Build history of the part. All positions in model axes, mm. A direction names the side the tool comes from. Round coordinates to 2 decimals unless told otherwise and drop trailing zeros. Loops run counter-clockwise (first coordinate to the right, second up) from the corner with the lowest first, then second, coordinate; pieces in that order, holes last.
Autodesk Inventor part; units mm, degrees
ref_plane "Work Plane2" through (0, 0, 11.8) normal (0, 0, 1) x (1, 0, 0)
ref_plane "Work Plane1" through (0, 0, 21.8) normal (0, 1, 0) x (0, 0, 1)
ref_plane "YZ Plane" through (0, 0, 0) normal (1, 0, 0) x (0, 1, 0)
sketch "Sketch1" plane through (0, 0, 0) normal (0, 0, 1) x (1, 0, 0)
  arc A0 (4.825, 0) -> (-4.825, 0) centre (0, 0) ccw
  line L0 (4.825, 0) -> (4.825, -3.775)
  line L1 (4.825, -3.775) -> (-4.825, -3.775)
  line L2 (-4.825, -3.775) -> (-4.825, 0)
  dimension "d0" = 9.65
  dimension "d2" = 3.775
  dimension "d3" = 9.65
extrude "Extrusion1" add sketch "Sketch1" along normal blind 8.8
sketch "Sketch2" plane through (0, 0, 8.8) normal (0, 0, 1) x (1, 0, 0)
  arc A0 (4.825, 0) -> (-4.825, 0) centre (0, 0) ccw
  circle A1 centre (0, 0) radius 4.825
extrude "Extrusion2" add sketch "Sketch2" along normal blind 13
ref_plane "Work Plane2" through (0, 0, 11.8) normal (0, 0, 1) x (1, 0, 0)
sketch "Sketch5" plane through (-4.825, -3.775, 0) normal (0, -1, 0) x (1, 0, 0)
  line L0 (1.82, 8.8) -> (7.83, 8.8)
  line L1 (0, 0) -> (0, 8.8)
  circle A0 centre (1.025, 4.2) radius 0.75
  circle A1 centre (8.625, 4.2) radius 0.75
  point P0 (4.825, 0)
  dimension "d15" = 1.5
  dimension "d17" = 1.5
  dimension "d18" = 4.6
  dimension "d19" = 4.6
  dimension "d20" = 7.6
  dimension "d21" = 1.025
extrude "Extrusion5" add sketch "Sketch5" along normal blind 3
sketch "Sketch6" plane through (0, 0, 0) normal (0, 0, -1) x (-1, 0, 0)
  arc A0 (4.825, 0) -> (-4.825, 0) centre (0, 0) ccw
  circle A1 centre (0, 0) radius 1.75
  dimension "d24" = 3.5
extrude "Extrusion6" add sketch "Sketch6" along normal blind 2
sketch "Sketch7" plane through (0, 0, -2) normal (0, 0, -1) x (-1, 0, 0)
  circle A0 centre (0, 0) radius 1.75
  line L0 (-0.375, 0.15) -> (-0.375, -0.15)
  line L1 (-0.375, -0.15) -> (0.375, -0.15)
  line L2 (0.375, -0.15) -> (0.375, 0.15)
  line L3 (0.375, 0.15) -> (-0.375, 0.15)
  dimension "d28" = 0.3
  dimension "d30" = 0.75
  dimension "d31" = 0.375
  dimension "d32" = 0.15
extrude "Extrusion7" add sketch "Sketch7" along normal blind 1.75 contours L3 L2 L1 L0
sketch "Sketch8" plane through (-0.375, -0.15, -2) normal (0, -1, 0) x (1, 0, 0)
  line L0 (0, 0) -> (0, -1.75)
  line L1 (0.75, -1.75) -> (0, -1.75)
  line L2 (0.75, 0) -> (0.75, -1.75)
  line L3 (0, -1.75) -> (0, -1.45)
  line L4 (0, -1.45) -> (0.75, -1.45)
  line L5 (0.75, -1.45) -> (0.75, -1.75)
  line L6 (0, -1.75) -> (0.75, -1.75)
  point P0 (0.375, 2)
  dimension "d35" = 0.3
  dimension "d36" = 0.75
extrude "Extrusion8" add sketch "Sketch8" along normal blind 6.625
fillet "Fillet1" radius 0.2 1 edges at (1.75, 0, -2)
fillet "Fillet2" radius 0.1 9 edges at (-0.375, -3.3125, -3.75) (0.375, -3.3125, -3.75) (-0.375, -3.4625, -3.45) (0, 0.15, -3.75) (-0.375, 0.15, -2.875) (-0.375, -0.15, -2.725) (0.375, 0.15, -2.875) (0.375, -0.15, -2.725) (0.375, -3.4625, -3.45)
ref_plane "Work Plane1" through (0, 0, 21.8) normal (0, 1, 0) x (0, 0, 1)
sketch "Sketch9" plane through (0, 0, 21.8) normal (0, 1, 0) x (0, 0, 1)
  circle A0 centre (-3, 0) radius 1
  line L0 (0, -4.825) -> (0, 4.825)
  line L1 (0, 0) -> (-8.1755, 0)
  point P0 (-21.8, 0)
  dimension "d42" = 2
  dimension "d44" = 3
  dimension "d45" = 0
extrude "Extrusion9" add sketch "Sketch9" along normal mid plane 11.02
sketch "Sketch3" plane through (0, 0, 21.8) normal (0, 0, 1) x (1, 0, 0)
  circle A0 centre (0, 0) radius 4.825
  circle A1 centre (0, 0) radius 4.25
  dimension "d8" = 8.5
extrude "Extrusion10" cut sketch "Sketch3" against normal blind 10 contours A1
sketch "Sketch4" plane through (0, 0, 11.8) normal (0, 0, 1) x (1, 0, 0)
  circle A0 centre (0, 0) radius 4.25
  circle A1 centre (0, 0) radius 0.5
  dimension "d12" = 1
extrude "Extrusion4" add sketch "Sketch4" along normal blind 10 contours A1
properties part number "0731000105"
(1) Slice it at D-D on y = -2.25. List the corners of the cut face in (x, z) (3 decimals).
Responses:
outline: (-4.825, 0) - (4.825, 0) - (4.825, 8.8) - (4.268, 8.8) - (4.268, 21.8) - (3.606, 21.8) - (3.606, 11.8) - (-3.606, 11.8) - (-3.606, 21.8) - (-4.268, 21.8) - (-4.268, 8.8) - (-4.825, 8.8) - close; (-0.375, -3.65) arc R0.1 ccw to (-0.275, -3.75) - (0.275, -3.75) arc R0.1 ccw to (0.375, -3.65) - (0.375, -3.55) arc R0.1 ccw to (0.275, -3.45) - (-0.275, -3.45) arc R0.1 ccw to (-0.375, -3.55) - close
(2) Pin check, flat tips, straight feed: P1, Ø1, axis at x = -0.5, z = 11.5, coming from the -Y side (3 decimals); P2, Ø0.9, axis at x = 0, y = 0.5, coming from the -Z side; P3, Ø2.5, axis at x = -1, y = 1.5, coming from the -Z side; P4, Ø1.6, axis at x = 0.5, z = 18.5, coming from the -Y side. Stop position of each tip, or through.
Responses:
P1: stops at y = -4.825
P2: stops at z = -3.75
P3: stops at z = -2
P4: stops at y = -5.51
(3) Slice it at B-B on z = 12.75. List the corners of the cut face in (x, y) (3 decimals), plus the area to 3 significant figures.
Responses:
outline: circle Ø9.65 at (0, 0); circle Ø1 at (0, 0); hole circle Ø8.5 at (0, 0)
area: 17.2 mm2
(4) Slice it at A-A on y = -5.75. List the corners of the cut face in (x, z) (3 decimals), plus the area to 3 significant figures.
Responses:
outline: circle Ø1.5 at (-3.8, 4.2); (-0.375, -3.65) arc R0.1 ccw to (-0.275, -3.75) - (0.275, -3.75) arc R0.1 ccw to (0.375, -3.65) - (0.375, -3.55) arc R0.1 ccw to (0.275, -3.45) - (-0.275, -3.45) arc R0.1 ccw to (-0.375, -3.55) - close; circle Ø1.5 at (3.8, 4.2)
area: 3.75 mm2
(5) Slice it at C-C on z = 4.2. List the corners of the cut face in (x, y) (3 decimals).
Responses:
outline: (-4.825, -3.775) - (-4.55, -3.775) - (-4.55, -6.775) - (-3.05, -6.775) - (-3.05, -3.775) - (3.05, -3.775) - (3.05, -6.775) - (4.55, -6.775) - (4.55, -3.775) - (4.825, -3.775) - (4.825, 0) arc R4.825 ccw to (-4.825, 0) - close
(6) Probe line 1 (Y direction, x = 0, z = 14.25) (3 decimals); line 2 (Z direction, x = 0, y = -1.25); line 3 (X direction, y = -0.25, z = 19.25). List the from-to ranges inside material, lowest first.
Responses:
line 1: y = -4.825 to -4.25, -0.5 to 0.5, 4.25 to 4.825
line 2: z = -3.75 to -3.45, -2 to 11.8
line 3: x = -4.82 to -4.24, -0.43 to 0.43, 4.24 to 4.82
(7) Pull direction Z, two halves, no side cores. Call faces 4 (the face through (4, -6.775, 4)), 5 (the face through (-4, -3, 8.8)), 6 (the face through (0, -4, 8.8)), 7 (the face through (0.383, 5.11, 19.724)): +Z half, -Z half, draft (parallel to the pull), parting line (faces both ways), or undercut.
Responses:
face 4: draft
face 5: +Z half
face 6: undercut
face 7: parting line
(8) Which spindle directions (+Z, -Z, +X, -X, +Y, -Y) get a long thin tool onto all of the face, cutting with end or side? Do faces 1 (the face through (0, 0, 21.8)), 2 (the face through (4.203, -5.254, 3.568)), 3 (the face through (-0.108, 0.488, 16.73)). Say none if no direction does.
Responses:
face 1: +Z, +X, -X, +Y, -Y
face 2: -Y
face 3: +Z
